Read the model definition and answer for the solid it produces. Units are mm, in the model's axes. A direction names the side the tool comes from. Coordinates: 2 decimals unless noted, no trailing zeros. Write each loop counter-clockwise with the first axis right and the second up, starting at its lowest first coordinate (ties: lowest second). Pieces come first, ordered by that corner, then holes.
(1) Determine the mould class of faces 3 (the flat face through (-62.003, 18, 4)), 4 (the cylindrical face through (18.7, 14.11, 6.03)), 5 (the flat face through (-25, 28.099, 4)), 6 (the cylindrical face through (-60.193, 10.187, 4.056)) for opening direction X: pulls with the +X half, pulls with the -X half, needs draft (parallel to the pull), parting line crosses it, or undercut.
(2) Which of the six approach directions +Z, -Z, +X, -X, +Y, -Y give full straight-line access (tool end or side, diameter ignored) to faces 1 (the flat face through (-15, 8.099, 4)), 2 (the cylindrical face through (39.91, 14.79, 6.03))?
(3) The part is cut by section B-B, the plane x = 35.5. Determine the outline of the cut face in (y, z).
(4) The part is cut by section D-D, the plane y = 30.5. Determine the outline of the cut face in (x, z), and give its area (3 significant figures).
(5) The part is cut by section A-A, the plane z = 7. State how many separate pieces and enclosed holes the cut face has, and give its area (3 significant figures).
(6) Given pin 1 (2 mm diameter, centred on y = 19, z = 5.5, fed in from +X); pin 2 (1.8 mm diameter, centred on x = 40.99, y = 28.1, fed in from +Z) (3 decimals); pin 3 (2.5 mm diameter, centred on x = -8.5, z = 3, fed in from +Y), each flat-ended and moving along its own axis, determine where each tip first touches the part or whether it passes through.
(7) The part is cut by section C-C, the plane z = 1. Determine the outline of the cut face in (x, y), and give its area (3 significant figures).
(8) Straight lines are drawn through the part: line 1 along Z through (x, y) = (22.5, 11.5); line 2 along Y through (x, z) = (-1.5, 3); line 3 along X through (y, z) = (36, 7.75). For each, find the intervals that lie inside material, in ascending order.
```python
from build123d import *

# Parameters (mm, degrees)
BOSS_EXTRU_1_DEPTH      = 8
ESQUISSE4_R             = 20
ESQUISSE4_R_2           = 15
ENL_V_MAT_EXTRU_2_DEPTH = 4
ESQUISSE5_W             = 16.42
ESQUISSE5_H             = 20
BOSS_EXTRU_2_DEPTH      = 8
ESQUISSE6_R             = 4
ESQUISSE6_R_2           = 1
ENL_V_MAT_EXTRU_3_DEPTH = 10
ESQUISSE7_R             = 1.5
ENL_V_MAT_EXTRU_4_DEPTH = 10


with BuildPart() as part:
    # Esquisse1 → Boss.-Extru.1 (new body)
    with BuildSketch(Plane.XY):
        with BuildLine():
            ThreePointArc((52.992232765, 28.099272116), (32.992232765, 48.099272116), (12.992232765, 28.099272116))
            Line((12.992232765, 28.099272116), (32.992232765, 28.099272116))
            Line((32.992232765, 28.099272116), (32.992232765, 8.099272116))
            ThreePointArc((32.992232765, 8.099272116), (47.134368389, 13.957136493), (52.992232765, 28.099272116))
        make_face()
        with BuildLine():
            Line((32.992232765, 28.099272116), (12.992232765, 28.099272116))
            ThreePointArc((12.992232765, 28.099272116), (18.850097141, 13.957136493), (32.992232765, 8.099272116))
            Line((32.992232765, 8.099272116), (32.992232765, 28.099272116))
        make_face()
        with BuildLine():
            Line((12.992232765, 28.099272116), (-45.58279523, 28.099272116))
            Line((-45.58279523, 28.099272116), (-45.58279523, 8.099272116))
            Line((-45.58279523, 8.099272116), (32.992232765, 8.099272116))
            ThreePointArc((32.992232765, 8.099272116), (18.850097141, 13.957136493), (12.992232765, 28.099272116))
        make_face()
    extrude(amount=BOSS_EXTRU_1_DEPTH)

    # Esquisse4 → Enlèv. mat.-Extru.2 (cut)
    with BuildSketch(Plane.XY.offset(8)):
        with Locations((32.992232765, 28.099272116)):
            Circle(ESQUISSE4_R)
        with Locations((32.992232765, 28.099272116)):
            Circle(ESQUISSE4_R_2, mode=Mode.SUBTRACT)
    extrude(amount=-ENL_V_MAT_EXTRU_2_DEPTH, mode=Mode.SUBTRACT)

    # Esquisse5 → Boss.-Extru.2 (add)
    with BuildSketch(Plane.XY.offset(8)):
        with Locations((-53.79279523, 18.099272116)):
            Rectangle(ESQUISSE5_W, ESQUISSE5_H)
    extrude(amount=-BOSS_EXTRU_2_DEPTH)

    # Esquisse6 → Enlèv. mat.-Extru.3 (cut)
    with BuildSketch(Plane.XY.offset(8)):
        with Locations((32.992232765, 28.099272116)):
            Circle(ESQUISSE6_R)
        with Locations((32.992232765, 36.099272116)):
            Circle(ESQUISSE6_R_2)
        with Locations((40.992232765, 28.099272116)):
            Circle(ESQUISSE6_R_2)
        with Locations((32.992232765, 20.099272116)):
            Circle(ESQUISSE6_R_2)
        with Locations((24.992232765, 28.099272116)):
            Circle(ESQUISSE6_R_2)
    extrude(amount=-ENL_V_MAT_EXTRU_3_DEPTH, mode=Mode.SUBTRACT)

    # Esquisse7 → Enlèv. mat.-Extru.4 (cut)
    with BuildSketch(Plane.XY.offset(8)):
        with Locations((-59.00279523, 25.099272116)):
            Circle(ESQUISSE7_R)
        with Locations((-59.00279523, 11.099272116)):
            Circle(ESQUISSE7_R)
    extrude(amount=-ENL_V_MAT_EXTRU_4_DEPTH, mode=Mode.SUBTRACT)


solid = part.part
```
Computed:
1. face 3: pulls with the -X half
1. face 4: undercut
1. face 5: needs draft
1. face 6: undercut
2. face 1: +Z, -Z, +X, -X, -Y
2. face 2: +Z
3. outline: (8.26, 0) - (24.98, 0) - (24.98, 8) - (13.31, 8) - (13.31, 4) - (8.26, 4) - close; (31.22, 0) - (47.94, 0) - (47.94, 4) - (42.89, 4) - (42.89, 8) - (31.22, 8) - close
4. outline: (13.14, 0) - (29.79, 0) - (29.79, 8) - (18.19, 8) - (18.19, 4) - (13.14, 4) - close; (36.19, 0) - (52.85, 0) - (52.85, 4) - (47.8, 4) - (47.8, 8) - (36.19, 8) - close
4. area: 226 mm2
5. separate pieces: 2
5. enclosed holes: 7
5. area: 2,220 mm2
6. pin 1: stops at x = 45.62
6. pin 2: passes through
6. pin 3: stops at y = 28.1
7. outline: (-62, 8.1) - (32.99, 8.1) arc R20 ccw (long way) to (12.99, 28.1) - (-62, 28.1) - close; hole circle Ø3 at (-59, 11.1); hole circle Ø3 at (-59, 25.1); hole circle Ø2 at (24.99, 28.1); hole circle Ø8 at (32.99, 28.1); hole circle Ø2 at (32.99, 20.1); hole circle Ø2 at (32.99, 36.1); hole circle Ø2 at (40.99, 28.1)
7. area: 2,770 mm2
8. line 1: z = 0 to 4
8. line 2: y = 8.1 to 28.1
8. line 3: x = 20.24 to 32, 33.99 to 45.74
